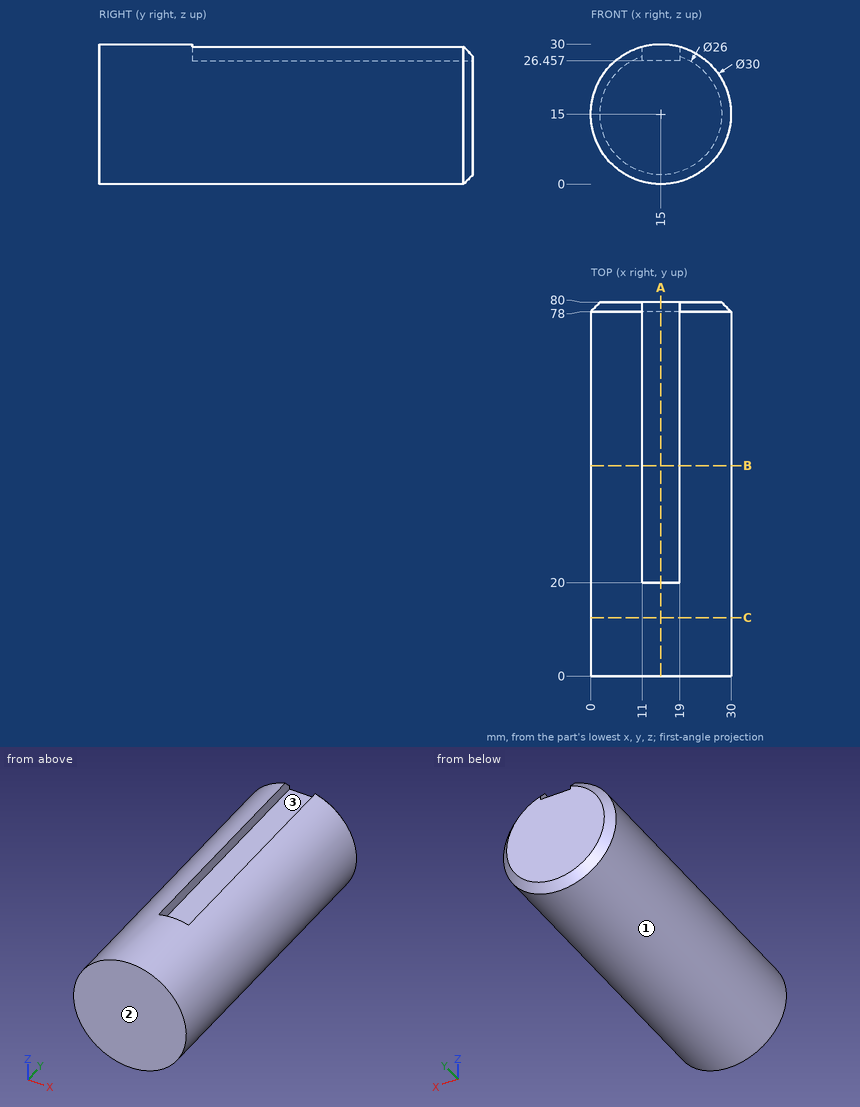
Can you work these out from the drawing? Everything is in mm from the part's minimum corner. Round coordinates to 2 decimals unless told otherwise and drop trailing zeros. Order: outer loops, then holes, each group sorted by start corner. A loop starts at its lowest first (then second) coordinate and runs counter-clockwise, first axis right, second up. Notation, with made-up numbers: M -30,75 L -16,75 A22 ccw -16,99 Z; hole C 83,-8.75 d5. An arc over 180 degrees is marked long. Answer as CSV lines item,"result".
Item 1: Please list where these lines run through material, in increasing order: L1, parallel to X at y = 35, z = 22.5; L2, parallel to X at y = 70, z = 26.5; L3, parallel to Z at x = 18.5, y = 28. Write a range as [from, to].
From the geometry:
L1,"[2.01, 27.99]"
L2,"[5.37, 11], [19, 24.63]"
L3,"[0.41, 26.46]"
Item 2: Imagine slicing it at C-C on y = 12.5. List the corners of the cut face in (x, z) for me.
From the geometry:
outline,"C 15,15 d30"
Item 3: For pin 1 (12 mm diameter, centred on x = 7, y = 13, fed in from -Z); pin 2 (6.5 mm diameter, centred on x = 15, y = 62.5, fed in from +Z); pin 3 (4 mm diameter, centred on x = 5.5, y = 70.5, fed in from +Z), each with a flat end and sliding along its axis, tell me the tip position at first contact or that it passes through.
From the geometry:
pin 1,"z = 0.13"
pin 2,"z = 26.46"
pin 3,"z = 27.99"
Item 4: We'd pull the mould along X, two halves only. Please class the marked faces 1, 2 and 3: +X half, -X half, draft (parallel to the pull), parting line (faces both ways), or undercut.
From the geometry:
face 1,"parting line"
face 2,"draft"
face 3,"undercut"
Item 5: Imagine slicing it at B-B on y = 45. List the corners of the cut face in (x, z) for me.
From the geometry:
outline,"M 11,26.46 L 11,29.46 A15 ccw long 19,29.46 L 19,26.46 Z"
Item 6: Imagine slicing it at A-A on x = 15. List the corners of the cut face in (y, z) for me, and give its area (3 significant figures).
From the geometry:
outline,"M 0,0 L 78,0 L 80,2 L 80,26.46 L 20,26.46 L 20,30 L 0,30 Z"
area,"2,190 mm2"
